The drawing under review shows one solid part. Ordinate dimensions are in mm from its lowest x, y, z. Coordinates: 2 decimals unless noted, no trailing zeros. Write each loop counter-clockwise with the first axis right and the second up, starting at its lowest first coordinate (ties: lowest second). Pieces come first, ordered by that corner, then holes. Notation, with made-up numbers: M 60.5,83 L 102.5,83 A35 cw 102.5,115 Z; hole C 46,68.5 d11. An arc over 180 degrees is marked long. Answer as CSV lines item,"result". Start each with the question number.
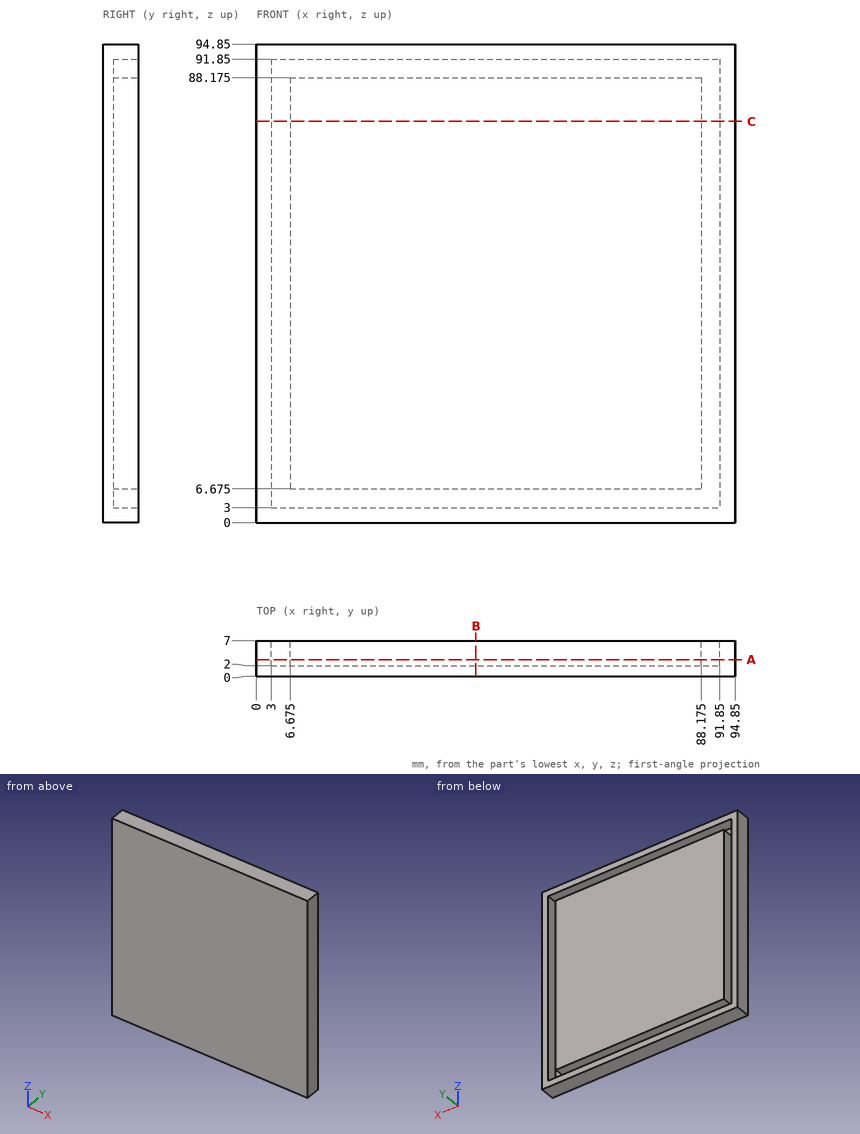
1) Take a section at C-C on z = 79.5. Give the boundary of the cut face in (x, y) (3 decimals).
2) Take a section at B-B on x = 43.5. Give the boundary of the cut face in (y, z) (3 decimals).
3) To check wall thickness, follow line 1 (X direction, y = 2.5, z = 12.5) (3 decimals); line 2 (X direction, y = 4.5, z = 6.5). State the ranges of each line that lie inside material, in increasing order. Write a range as [from, to].
4) Take a section at A-A on y = 3.25. Give the boundary of the cut face in (x, z) (3 decimals).
Results:
1,outline,"M 0,0 L 94.85,0 L 94.85,7 L 91.85,7 L 91.85,2 L 88.175,2 L 88.175,7 L 6.675,7 L 6.675,2 L 3,2 L 3,7 L 0,7 Z"
2,outline,"M 0,0 L 7,0 L 7,3 L 2,3 L 2,6.675 L 7,6.675 L 7,88.175 L 2,88.175 L 2,91.85 L 7,91.85 L 7,94.85 L 0,94.85 Z"
3,line 1,"x = [0, 3], [6.675, 88.175], [91.85, 94.85]"
3,line 2,"x = [0, 3], [91.85, 94.85]"
4,outline,"M 0,0 L 94.85,0 L 94.85,94.85 L 0,94.85 Z; M 6.675,6.675 L 88.175,6.675 L 88.175,88.175 L 6.675,88.175 Z; hole M 3,3 L 91.85,3 L 91.85,91.85 L 3,91.85 Z"
